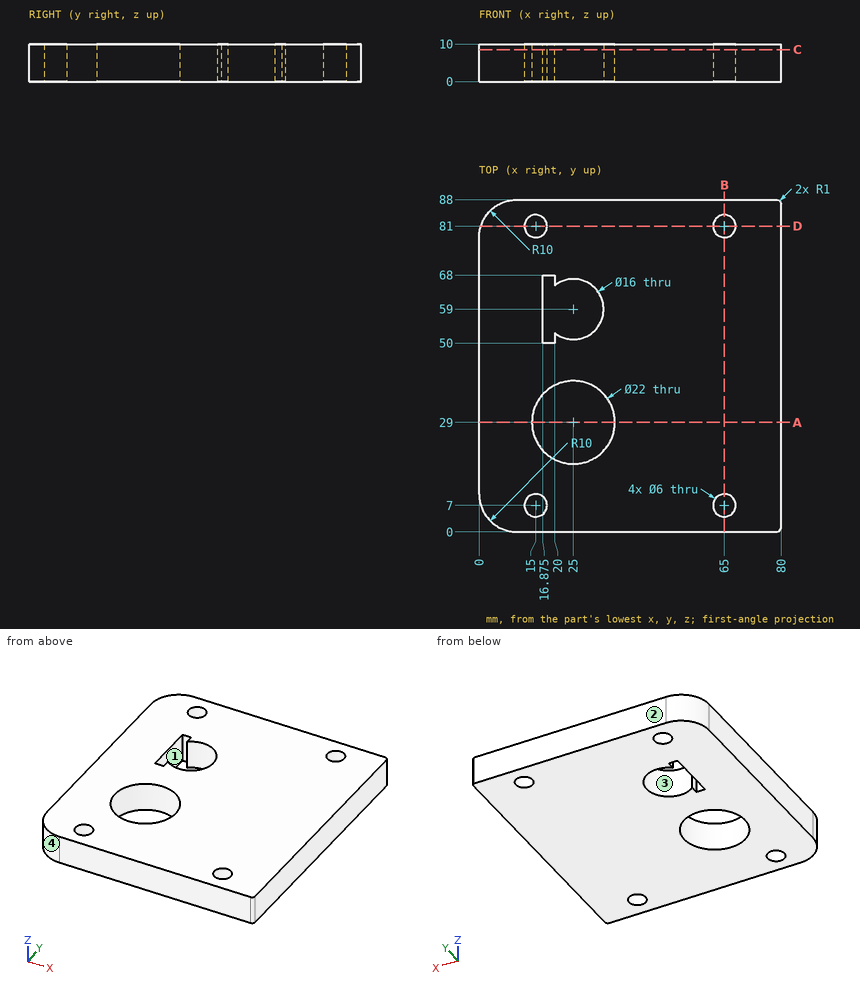
Could you check a few things on this drawing? It's one solid part, dimensions in mm from its lowest x, y, z. Round coordinates to 2 decimals unless told otherwise and drop trailing zeros. Order: outer loops, then holes, each group sorted by start corner. A loop starts at its lowest first (then second) coordinate and runs counter-clockwise, first axis right, second up.
Q1. I'm going to push flat-ended pins straight in: P1, Ø9.5, axis at x = 25, y = 59, coming from the -Z side; P2, Ø1.5, axis at y = 58, z = 2.5, coming from the -X side. Where does each tip first touch, or does it pass through?
Geometry says:
P1: passes through
P2: stops at x = 0
Q2. Thinking about a two-plate mould opening in Y: for the marked faces 1, 2, 3 and 4, which applies, released by +Y, released by -Y, zero draft, split by the parting line, or undercut?
Geometry says:
face 1: undercut
face 2: released by +Y
face 3: undercut
face 4: released by -Y
Q3. Imagine slicing it at C-C, the plane z = 8.5. List the corners of the cut face in (x, y) for me (3 decimals).
Geometry says:
outline: (0, 10) arc R10 ccw to (10, 0) - (79, 0) arc R1 ccw to (80, 1) - (80, 87) arc R1 ccw to (79, 88) - (10, 88) arc R10 ccw to (0, 78) - close; hole circle Ø6 at (15, 7); hole circle Ø6 at (15, 81); hole circle Ø22 at (25, 29); hole (16.875, 50) - (20, 50) - (20, 52.755) arc R8 ccw (long way) to (20, 65.245) - (20, 68) - (16.875, 68) - close; hole circle Ø6 at (65, 7); hole circle Ø6 at (65, 81)
Q4. Imagine slicing it at B-B, the plane x = 65. List the corners of the cut face in (y, z) for me, then the cut area to 3 significant figures.
Geometry says:
outline: (0, 0) - (4, 0) - (4, 10) - (0, 10) - close; (10, 0) - (78, 0) - (78, 10) - (10, 10) - close; (84, 0) - (88, 0) - (88, 10) - (84, 10) - close
area: 760 mm2
Q5. Imagine slicing it at A-A, the plane y = 29. List the corners of the cut face in (x, z) for me.
Geometry says:
outline: (0, 0) - (14, 0) - (14, 10) - (0, 10) - close; (36, 0) - (80, 0) - (80, 10) - (36, 10) - close
Q6. Imagine slicing it at D-D, the plane y = 81. List the corners of the cut face in (x, z) for me.
Geometry says:
outline: (0.46, 0) - (12, 0) - (12, 10) - (0.46, 10) - close; (18, 0) - (62, 0) - (62, 10) - (18, 10) - close; (68, 0) - (80, 0) - (80, 10) - (68, 10) - close
Q7. Please list where these lines run through material, in increasing order: probe 1 along Y at (x, z) = (25, 6); probe 2 along X at (y, z) = (5, 4.5); probe 3 along Y at (x, z) = (21, 3.25).
Geometry says:
probe 1: y = 0 to 18, 40 to 51, 67 to 88
probe 2: x = 1.34 to 12.76, 17.24 to 62.76, 67.24 to 80
probe 3: y = 0 to 18.75, 39.25 to 52.07, 65.93 to 88
